```python
from build123d import *

# Parameters (mm, degrees)
F0_W     = 70
F0_H     = 70
F0_R     = 27.5
F1_DEPTH = 50
F2_W     = 20
F2_H     = 15
F3_DEPTH = 25
F4_R     = 4


with BuildPart() as f1:
    # F0 (on Top) → F1 (new body)
    with BuildSketch(Plane.XY):
        Rectangle(F0_W, F0_H)
        Circle(F0_R, mode=Mode.SUBTRACT)
    extrude(amount=F1_DEPTH)

    # F2 (on face) → F3 (cut)
    with BuildSketch(Plane.XZ.offset(35)):
        with Locations((0, 25)):
            Rectangle(F2_W, F2_H)
    extrude(amount=-F3_DEPTH, mode=Mode.SUBTRACT)

    # F4
    f4_edges = [f1.edges().sort_by_distance(p)[0] for p in [
        (-10, -30.308688, 32.5),
        (10, -30.308688, 32.5),
        (10, -30.308688, 17.5),
        (-10, -30.308688, 17.5),
    ]]
    fillet(f4_edges, radius=F4_R)


solid = f1.part
```
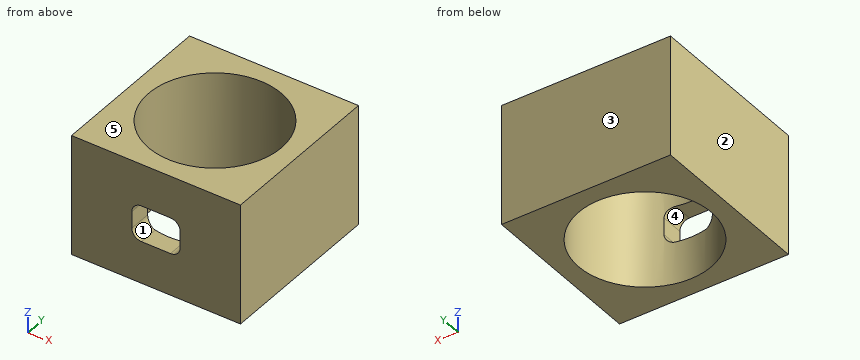
Input: part model. Units: mm. Frame: model coordinates. Face numbers are marked on the shaded views. A direction names the side the tool comes from. Round coordinates to 2 decimals unless told otherwise and drop trailing zeros. Loops run counter-clockwise (first coordinate to the right, second up) from the corner with the lowest first, then second, coordinate; pieces in that order, holes last.
1) Set-up query: the marked faces 1 and 2. Return all of +Z, -Z, +X, -X, +Y, -Y with unobstructed straight access to the full face (end or side cutting, diameter ignored); none if empty.
Ans:
face 1: -Y
face 2: +Z, -Z, -X, +Y, -Y
2) Section query A-A on y = 0. Return the cut outline in (x, z), plus the area to 3 significant figures.
Ans:
outline: (-35, 0) - (-27.5, 0) - (-27.5, 50) - (-35, 50) - close; (27.5, 0) - (35, 0) - (35, 50) - (27.5, 50) - close
area: 750 mm2
3) Material intervals for line 1 (X direction, y = 1, z = 40.5); line 2 (Y direction, x = 0, z = 39); line 3 (X direction, y = 23.5, z = 31), sorted ascending.
Ans:
line 1: x = -35 to -27.48, 27.48 to 35
line 2: y = -35 to -27.5, 27.5 to 35
line 3: x = -35 to -14.28, 14.28 to 35
4) Section query B-B on x = 0. Return the cut outline in (y, z).
Ans:
outline: (-35, 0) - (-27.5, 0) - (-27.5, 17.5) - (-35, 17.5) - close; (-35, 32.5) - (-27.5, 32.5) - (-27.5, 50) - (-35, 50) - close; (27.5, 0) - (35, 0) - (35, 50) - (27.5, 50) - close
5) Section query D-D on y = 16.5. Return the cut outline in (x, z), plus the area to 3 significant figures.
Ans:
outline: (-35, 0) - (-22, 0) - (-22, 50) - (-35, 50) - close; (22, 0) - (35, 0) - (35, 50) - (22, 50) - close
area: 1,300 mm2
6) Pull-direction query (Z, two-part tool) for the marked faces 3, 4 and 5; classes: released by +Z, released by -Z, zero draft, split by the parting line, or undercut.
Ans:
face 3: zero draft
face 4: undercut
face 5: released by +Z
7) Section query C-C on z = 44. Return the cut outline in (x, y), plus the area to 3 significant figures.
Ans:
outline: (-35, -35) - (35, -35) - (35, 35) - (-35, 35) - close; hole circle Ø55 at (0, 0)
area: 2,520 mm2
8) Pin query (flat end, axial travel): pin 1 (6.5 mm diameter, centred on x = -1.5, y = -30, fed in from -Z). Return the tip coordinate at first contact, or that it passes through.
Ans:
pin 1: stops at z = 0
